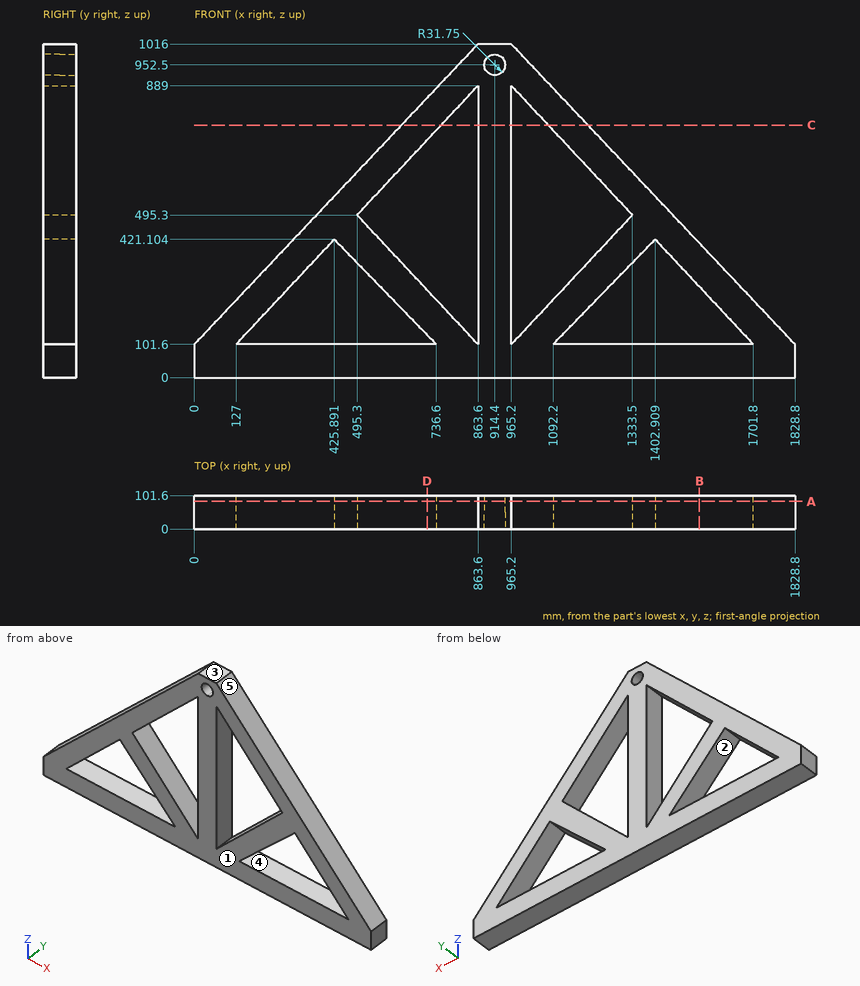
Design review of the part shown in the three views and the two pictorial views. Dimensions are in mm from the part's minimum x, y and z. A direction names the side the tool comes from. Round coordinates to 2 decimals unless told otherwise and drop trailing zeros. Write each loop counter-clockwise with the first axis right and the second up, starting at its lowest first coordinate (ties: lowest second). Pieces come first, ordered by that corner, then holes. Notation, with made-up numbers: (2, 55.5) - (48, 55.5) arc R28 ccw to (48, 85.5) - close; hole circle Ø8 at (11.5, -29.5). An arc over 180 degrees is marked (long way). Answer as CSV lines item,"result". Start each with the question number.
(1) Add section C-C, the plane z = 769. State the section outline as (x, y) points.
(2) For line 1 (X direction, y = 24, z = 357) (1 decimal); line 2 (X direction, y = 43.5, z = 151) (1 decimal); line 3 (Z direction, x = 528.5, y = 11), list the stretches that pass through material, from the lowest coordinate up.
(3) Add section B-B, the plane x = 1537.5. State the section outline as (y, z) points (1 decimal).
(4) Add section D-D, the plane x = 708.5. State the section outline as (y, z) points (1 decimal), plus the area to 3 significant figures.
(5) Machinability: for the marked faces 4 and 5, which of the approach directions +Z, -Z, +X, -X, +Y, -Y give a long, thin tool a straight path to every point of the face, cutting with its end or side? Answer none if there is none.
(6) For pin 1 (1 mm diameter, centred on x = 914.5, y = 86.5, fed in from -Z); pin 2 (4 mm diameter, centred on x = 975.5, y = 49, fed in from +Z); pin 3 (2 mm diameter, centred on x = 634, y = 54.5, fed in from +Z); pin 4 (4 mm diameter, centred on y = 27.5, z = 328, fed in from -X), all flat-tipped, find the tip position at first contact; note any pin that passes through.
(7) Add section A-A, the plane y = 84. State how many separate pieces and enclosed holes the cut face has, plus the area to 3 significant figures.
(8) Mouldability with a two-part tool opening along Z and no side actions: class the marked faces 1, 2 and 3 as +Z half, -Z half, draft (parallel to the pull), parting line (faces both ways), or undercut.
From the geometry:
1,outline,"(630.32, 0) - (751.34, 0) - (751.34, 101.6) - (630.32, 101.6) - close; (863.6, 0) - (965.2, 0) - (965.2, 101.6) - (863.6, 101.6) - close; (1077.46, 0) - (1198.48, 0) - (1198.48, 101.6) - (1077.46, 101.6) - close"
2,line 1,"x = 241.2 to 365.9, 488.2 to 624.7, 863.6 to 965.2, 1204.1 to 1340.6, 1462.9 to 1587.6"
2,line 2,"x = 46.7 to 173.2, 688.6 to 817.4, 863.6 to 965.2, 1011.4 to 1140.2, 1655.6 to 1782.1"
2,line 3,"z = 0 to 101.6, 315.59 to 459.81, 530.79 to 661.19"
3,outline,"(0, 0) - (101.6, 0) - (101.6, 101.6) - (0, 101.6) - close; (0, 277.2) - (101.6, 277.2) - (101.6, 410) - (0, 410) - close"
4,outline,"(0, 0) - (101.6, 0) - (101.6, 101.6) - (0, 101.6) - close; (0, 130.5) - (101.6, 130.5) - (101.6, 267.4) - (0, 267.4) - close; (0, 723.2) - (101.6, 723.2) - (101.6, 851.8) - (0, 851.8) - close"
4,area,"37,300 mm²"
5,face 4,"+Y, -Y"
5,face 5,"+Z, +X, +Y, -Y"
6,pin 1,"stops at z = 0"
6,pin 2,"stops at z = 1007.21"
6,pin 3,"stops at z = 773.95"
6,pin 4,"stops at x = 211.93"
7,separate pieces,"1"
7,enclosed holes,"5"
7,area,"580,000 mm²"
8,face 1,"draft"
8,face 2,"undercut"
8,face 3,"+Z half"
